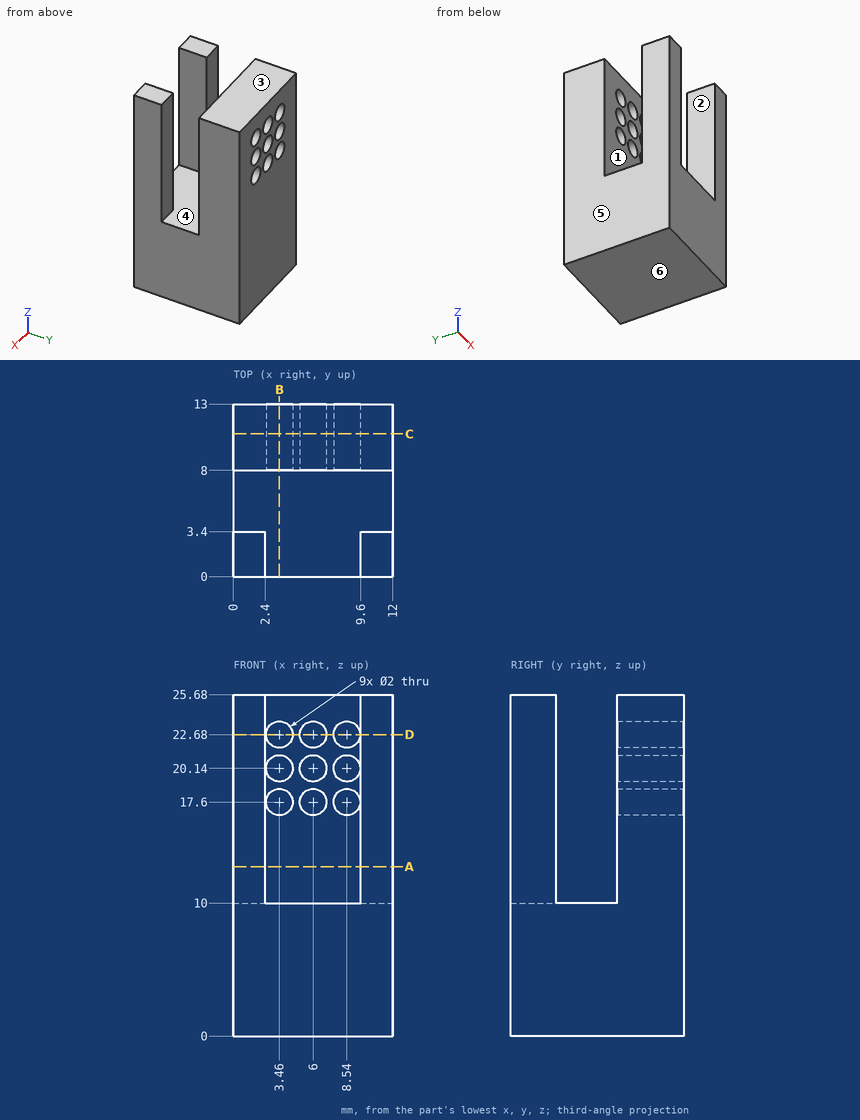
Drawing for the job (mm, zero at the part's lowest x, y, z). A direction names the side the tool comes from. Coordinates: 2 decimals unless noted, no trailing zeros. Order: outer loops, then holes, each group sorted by start corner. A loop starts at its lowest first (then second) coordinate and runs counter-clockwise, first axis right, second up.
Item 1: 3-axis set-ups, long thin cutter, end or side, ignore diameter. For the marked faces 1, 2 and 3: which of +Z, -Z, +X, -X, +Y, -Y reach the whole face in a straight line?
Check sheet entries:
face 1: +Z, +X, -X
face 2: +Z, -Y
face 3: +Z, +X, -X, +Y, -Y
Item 2: Two-plate mould, pull along X, no slides. Class the marked faces 4, 5 and 6: +X half, -X half, draft (parallel to the pull), parting line (faces both ways), or undercut.
Check sheet entries:
face 4: undercut
face 5: -X half
face 6: draft
Item 3: Band-saw the part on C-C on y = 10.75. Give the number of separate pieces and of enclosed holes in the cut face, plus the area to 3 significant figures.
Check sheet entries:
separate pieces: 1
enclosed holes: 9
area: 280 mm2
Item 4: Band-saw the part on B-B on x = 3.46. List the corners of the cut face in (y, z), plus the area to 3 significant figures.
Check sheet entries:
outline: (0, 0) - (13, 0) - (13, 16.6) - (8, 16.6) - (8, 10) - (0, 10) - close; (8, 18.6) - (13, 18.6) - (13, 19.14) - (8, 19.14) - close; (8, 21.14) - (13, 21.14) - (13, 21.68) - (8, 21.68) - close; (8, 23.68) - (13, 23.68) - (13, 25.68) - (8, 25.68) - close
area: 178 mm2
Item 5: Band-saw the part on A-A on z = 12.75. List the corners of the cut face in (x, y).
Check sheet entries:
outline: (0, 0) - (2.4, 0) - (2.4, 3.4) - (0, 3.4) - close; (0, 8) - (12, 8) - (12, 13) - (0, 13) - close; (9.6, 0) - (12, 0) - (12, 3.4) - (9.6, 3.4) - close
Item 6: Band-saw the part on D-D on z = 22.68. List the corners of the cut face in (x, y), plus the area to 3 significant figures.
Check sheet entries:
outline: (0, 0) - (2.4, 0) - (2.4, 3.4) - (0, 3.4) - close; (0, 8) - (2.46, 8) - (2.46, 13) - (0, 13) - close; (4.46, 8) - (5, 8) - (5, 13) - (4.46, 13) - close; (7, 8) - (7.54, 8) - (7.54, 13) - (7, 13) - close; (9.54, 8) - (12, 8) - (12, 13) - (9.54, 13) - close; (9.6, 0) - (12, 0) - (12, 3.4) - (9.6, 3.4) - close
area: 46.3 mm2
Item 7: Pin check, flat tips, straight feed: pin 1 Ø2.5 at (x, z) = (6, 17.6) entering from -Y; pin 2 Ø1.2 at (x, z) = (3.46, 22.68) entering from +Y. Stop position of each tip, or through.
Check sheet entries:
pin 1: stops at y = 8
pin 2: passes through
Item 8: Drill centre lines: L1, parallel to X at y = 11.4, z = 17.6; L2, parallel to Y at x = 2, z = 19.5; L3, parallel to Z at x = 3.5, y = 12.25. Where is each one in solid material? Low to high.
Check sheet entries:
L1: x = 0 to 2.46, 4.46 to 5, 7 to 7.54, 9.54 to 12
L2: y = 0 to 3.4, 8 to 13
L3: z = 0 to 16.6, 18.6 to 19.14, 21.14 to 21.68, 23.68 to 25.68
